For this review, take the finished solid that the model builds, in its own axes (mm). Give positions to 0.01 mm unless a question says otherwise; leave off trailing zeros. Loops run counter-clockwise (first coordinate to the right, second up) from the corner with the lowest first, then second, coordinate; pieces in that order, holes last. Notation, with made-up numbers: (-31.75, 62.5) - (0.25, 62.5) arc R31 ccw to (0.25, 93.5) - close; hole circle Ø11 at (10, 64). An arc over 180 degrees is marked (long way). Put each result on its own line as item: value. Start each with the question number.
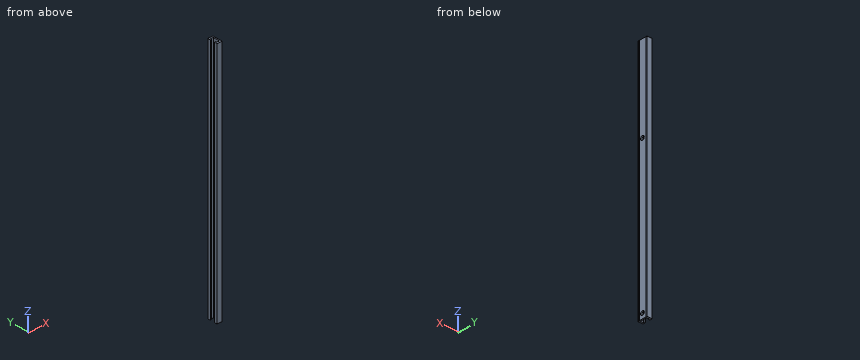
from build123d import *

# Parameters (mm, degrees)
F1_DEPTH = 457.2
F3_D     = 7.62
F3_DEPTH = 25.4


with BuildPart() as f1:
    # F0 (on Top) → F1 (new body)
    with BuildSketch(Plane.XY):
        with BuildLine():
            Line((-4.8895, -9.525), (4.8895, -9.525))
            Line((4.8895, -9.525), (4.8895, -6.861627))
            ThreePointArc((4.8895, -6.861627), (4.593677, -6.366351), (4.8895, -5.871076))
            Line((4.8895, -5.871076), (4.8895, 5.871076))
            ThreePointArc((4.8895, 5.871076), (4.593677, 6.366351), (4.8895, 6.861627))
            Line((4.8895, 6.861627), (4.8895, 9.525))
            Line((4.8895, 9.525), (-4.8895, 9.525))
            Line((-4.8895, 9.525), (-4.8895, 4.445))
            Line((-4.8895, 4.445), (-2.54, 4.445))
            Line((-2.54, 4.445), (-2.54, 6.35))
            Line((-2.54, 6.35), (2.54, 6.35))
            Line((2.54, 6.35), (2.54, -6.35))
            Line((2.54, -6.35), (-2.54, -6.35))
            Line((-2.54, -6.35), (-2.54, -4.445))
            Line((-2.54, -4.445), (-4.8895, -4.445))
            Line((-4.8895, -4.445), (-4.8895, -9.525))
        make_face()
    extrude(amount=F1_DEPTH)

    # F3
    with Locations(Plane.YZ.offset(4.8895)):
        with Locations((0, 9.525), (0, 295.275)):
            Hole(F3_D / 2, depth=F3_DEPTH)


solid = f1.part
1) Take a section at B-B on x = 0. State the section outline as (y, z) points (3 decimals), and give its area (3 significant figures).
2) Take a section at A-A on y = 0. State the section outline as (x, z) points (1 decimal).
3) Wall thickness on probe 1 along Z at (x, y) = (3.3, 0) (3 decimals); probe 2 along Y at (x, z) = (-4.5, 358) (3 decimals); probe 3 along Y at (x, z) = (-0.75, 168.5) (3 decimals): over which ranges is each line inside the solid? List them lowest first.
4) Insertion check: P1, Ø4.5, axis at y = 0, z = 295.275, coming from the +X side. The pin has a flat end and moves straight along its axis. Give the tip position at first contact, or say it passes through.
Answers follow:
1. outline: (-9.525, 0) - (-6.35, 0) - (-6.35, 457.2) - (-9.525, 457.2) - close; (6.35, 0) - (9.525, 0) - (9.525, 457.2) - (6.35, 457.2) - close
1. area: 2,900 mm2
2. outline: (2.5, 0) - (4.9, 0) - (4.9, 5.7) - (2.5, 5.7) - close; (2.5, 13.3) - (4.9, 13.3) - (4.9, 291.5) - (2.5, 291.5) - close; (2.5, 299.1) - (4.9, 299.1) - (4.9, 457.2) - (2.5, 457.2) - close
3. probe 1: 0 to 5.715, 13.335 to 291.465, 299.085 to 457.2
3. probe 2: -9.525 to -4.445, 4.445 to 9.525
3. probe 3: -9.525 to -6.35, 6.35 to 9.525
4. P1: through
